```python
from build123d import *

# Parameters (mm, degrees)
ESQUISSE1_W             = 60
ESQUISSE1_H             = 40
BOSS_EXTRU_1_DEPTH      = 4
ESQUISSE2_W             = 4.4
ESQUISSE2_H             = 7.4
ESQUISSE2_H_2           = 10.4
ENL_V_MAT_EXTRU_1_DEPTH = 37.276714294
ENL_V_MAT_EXTRU_2_DEPTH = 37.276714294


with BuildPart() as part:
    # Esquisse1 → Boss.-Extru.1 (new body)
    with BuildSketch(Plane.XY):
        Rectangle(ESQUISSE1_W, ESQUISSE1_H)
    extrude(amount=BOSS_EXTRU_1_DEPTH)

    # Esquisse2 → Enlèv. mat.-Extru.1 (cut, through all)
    with BuildSketch(Plane(origin=(0, 0, 0), x_dir=(-1, 0, 0), z_dir=(0, 0, -1))):
        with Locations((-28, -16.5)):
            Rectangle(ESQUISSE2_W, ESQUISSE2_H)
        with Locations((-28, 16.5)):
            Rectangle(ESQUISSE2_W, ESQUISSE2_H)
        with Locations((-28, 0)):
            Rectangle(ESQUISSE2_W, ESQUISSE2_H_2)
        with Locations((28, 0)):
            Rectangle(ESQUISSE2_W, ESQUISSE2_H_2)
        with Locations((28, 16.5)):
            Rectangle(ESQUISSE2_W, ESQUISSE2_H)
        with Locations((28, -16.5)):
            Rectangle(ESQUISSE2_W, ESQUISSE2_H)
    extrude(amount=-ENL_V_MAT_EXTRU_1_DEPTH, mode=Mode.SUBTRACT)

    # Esquisse3 → Enlèv. mat.-Extru.2 (cut, through all)
    with BuildSketch(Plane(origin=(0, 0, 0), x_dir=(-1, 0, 0), z_dir=(0, 0, -1))):
        Polygon((-25.8, -2.1), (-25.8, 2.1), (-24, 2.1), (-24, 3.5), (-20.8, 3.5), (-20.8, 2.1), (-14.8, 2.1), (-14.8, -2.1), (-20.8, -2.1), (-20.8, -3.5), (-24, -3.5), (-24, -2.1), align=None)
        Polygon((25.8, -2.1), (24, -2.1), (24, -3.5), (20.8, -3.5), (20.8, -2.1), (14.8, -2.1), (14.8, 2.1), (20.8, 2.1), (20.8, 3.5), (24, 3.5), (24, 2.1), (25.8, 2.1), align=None)
    extrude(amount=-ENL_V_MAT_EXTRU_2_DEPTH, mode=Mode.SUBTRACT)


solid = part.part
```
Can you work these out from the model? Positions are in its coordinate system, mm. A direction names the side the tool comes from. Give positions to 0.01 mm unless a question says otherwise; leave off trailing zeros. Loops run counter-clockwise (first coordinate to the right, second up) from the corner with the lowest first, then second, coordinate; pieces in that order, holes last. Notation, with made-up numbers: M -19.75,-12.5 L -3.75,-12.5 A23 cw -3.75,17.5 Z; hole C 36.5,89.5 d8. An arc over 180 degrees is marked long. One line per question, with ' | ' between items. Start each with the question number.
Q1. If we section it at A-A (x = 18.5): Please give me the cut outline in (y, z), plus the area to 3 significant figures.
Q2. If we section it at C-C (y = 4.5): Please give me the cut outline in (x, z), plus the area to 3 significant figures.
Q3. If we section it at B-B (x = 26.5): Please give me the cut outline in (y, z), plus the area to 3 significant figures.
Q4. If I drill on line 1 (X direction, y = -2.5, z = 3.3); line 2 (Y direction, x = 15, z = 0.35); line 3 (Y direction, x = -28, z = 1.9), over which ranges is the centre line in solid material (lowest first)? Write a range as from..to.
Q5. If we mould it in two halves opening along Y, with no side actions, what happens to faces 1 (the flat face through (22, -3.5, 2)), 2 (the flat face through (25, -2.1, 2)), 3 (the flat face through (0, 20, 2)), 4 (the flat face through (-25.8, 16, 2))? For each: +Y half, -Y half, draft (parallel to the pull), parting line (faces both ways), or undercut.
Q6. For faces 5 (the flat face through (22, 3.5, 2)), 6 (the flat face through (28, -12.8, 2)), 7 (the flat face through (-28, -12.8, 2)), which set-ups out of +Z, -Z, +X, -X, +Y, -Y let a thin tool reach every point of the face, with its end or its side?
Q7. For pin 1 Ø4 at (x, y) = (-20.5, -6.5) entering from -Z; pin 2 Ø2 at (y, z) = (-1, 3) entering from +X; pin 3 Ø1.2 at (y, z) = (-17.5, 3) entering from +X; pin 4 Ø1.2 at (x, z) = (28, 2.5) entering from -Y, each with a flat end and sliding along its axis, tell me the tip position at first contact or that it passes through.
Computed:
1) outline: M -20,0 L -2.1,0 L -2.1,4 L -20,4 Z; M 2.1,0 L 20,0 L 20,4 L 2.1,4 Z | area: 143 mm²
2) outline: M -25.8,0 L 25.8,0 L 25.8,4 L -25.8,4 Z | area: 206 mm²
3) outline: M -12.8,0 L -5.2,0 L -5.2,4 L -12.8,4 Z; M 5.2,0 L 12.8,0 L 12.8,4 L 5.2,4 Z | area: 60.8 mm²
4) line 1: x = -25.8..-24, -20.8..20.8, 24..25.8 | line 2: y = -20..-2.1, 2.1..20 | line 3: y = -12.8..-5.2, 5.2..12.8
5) face 1: undercut | face 2: undercut | face 3: +Y half | face 4: draft
6) face 5: +Z, -Z | face 6: +Z, -Z, +X, -Y | face 7: +Z, -Z, -X, -Y
7) pin 1: stops at z = 0 | pin 2: stops at x = 14.8 | pin 3: stops at x = 25.8 | pin 4: stops at y = -12.8
